For this review, use the dimensioned drawing (mm, ordinates from the lowest corner) and the shaded views. Round coordinates to 2 decimals unless told otherwise and drop trailing zeros. Order: outer loops, then holes, each group sorted by start corner. A loop starts at its lowest first (then second) coordinate and runs counter-clockwise, first axis right, second up. Notation, with made-up numbers: (11.5, 14.25) - (58.5, 14.25) arc R20 ccw to (58.5, 51.25) - close; hole circle Ø1 at (83.25, 7.5). An arc over 180 degrees is marked (long way). Write item = value, one per line.
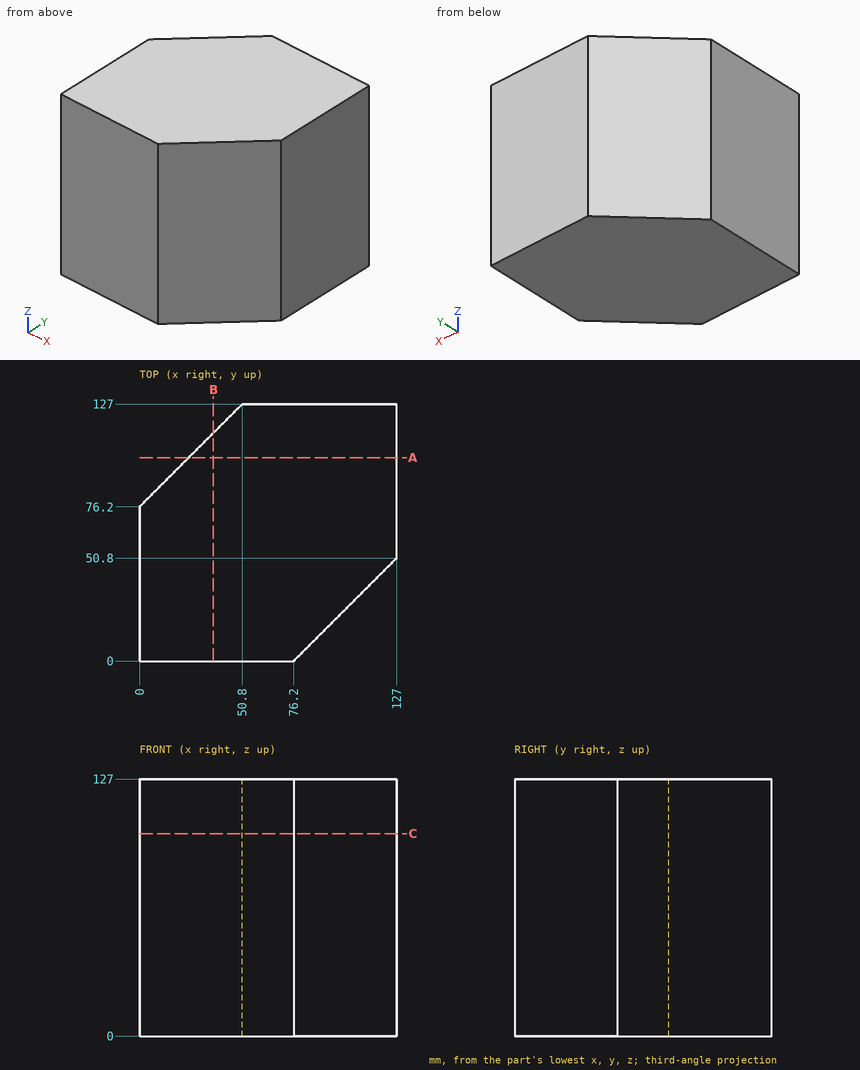
1) We need section C-C on z = 100. Write out the cut boundary in (x, y), and give its area (3 significant figures).
Findings:
outline = (0, 0) - (76.2, 0) - (127, 50.8) - (127, 127) - (50.8, 127) - (0, 76.2) - close
area = 13,500 mm^2
2) Clearance check with flat-ended pins moving along their axes: pin 1 Ø2 at (x, z) = (113.5, 104) entering from -Y; pin 2 Ø5 at (y, z) = (21.5, 37.5) entering from +X. State where each tip first meets the part, or that it passes through.
Findings:
pin_1 = 36.3
pin_2 = 100.2
3) We need section A-A on y = 100.5. Write out the cut boundary in (x, z).
Findings:
outline = (24.3, 0) - (127, 0) - (127, 127) - (24.3, 127) - close
4) To check wall thickness, follow L1, parallel to X at y = 12.5, z = 113.5; L2, parallel to X at y = 102, z = 11.5; L3, parallel to Y at x = 32, z = 35.5. State the ranges of each line that lie inside material, in increasing order. Write a range as from..to.
Findings:
L1 = 0..88.7
L2 = 25.8..127
L3 = 0..108.2
5) We need section B-B on x = 36.5. Write out the cut boundary in (y, z).
Findings:
outline = (0, 0) - (112.7, 0) - (112.7, 127) - (0, 127) - close
